```python
from build123d import *

# Parameters (mm, degrees)
F0_R     = 2.032
F0_R_2   = 2.027946
F0_R_3   = 6.35
F1_DEPTH = 6.35


with BuildPart() as f1:
    # F0 (on Top) → F1 (new body)
    with BuildSketch(Plane.XY):
        with BuildLine():
            Line((-170.272195, -49.641607), (-163.925477, -49.641607))
            ThreePointArc((-163.925477, -49.641607), (-140.909058, -31.963569), (-132.186283, -4.28358))
            Line((-132.186283, -4.28358), (-132.186283, -2.299813))
            Line((-132.186283, -2.299813), (-132.186283, 29.155357))
            ThreePointArc((-132.186283, 29.155357), (-133.837078, 32.141068), (-137.035743, 33.327715))
            Line((-137.035743, 33.327715), (-148.047195, 33.327715))
            Line((-148.047195, 33.327715), (-148.047195, 34.918903))
            Line((-148.047195, 34.918903), (-186.147195, 34.918903))
            Line((-186.147195, 34.918903), (-186.147195, 33.327715))
            Line((-186.147195, 33.327715), (-197.693917, 33.327715))
            Line((-197.693917, 33.327715), (-198.24493, 33.327715))
            ThreePointArc((-198.24493, 33.327715), (-201.203656, 31.805681), (-202.114563, 28.605541))
            Line((-202.114563, 28.605541), (-202.114563, 13.871952))
            Line((-202.114563, 13.871952), (-246.486589, 13.871952))
            Line((-246.486589, 13.871952), (-246.486589, -49.641607))
            Line((-246.486589, -49.641607), (-240.805238, -49.641607))
            Line((-240.805238, -49.641607), (-170.272195, -49.641607))
        make_face()
        with Locations((-234.114588, -44.87283)):
            Circle(F0_R, mode=Mode.SUBTRACT)
        with Locations((-167.098836, -46.955632)):
            Circle(F0_R, mode=Mode.SUBTRACT)
        with Locations((-167.098836, -41.466439)):
            Circle(F0_R_2, mode=Mode.SUBTRACT)
        with Locations((-233.186065, -3.547357)):
            Circle(F0_R_3, mode=Mode.SUBTRACT)
        with Locations((-197.969424, 21.535357)):
            Circle(F0_R, mode=Mode.SUBTRACT)
        with Locations((-197.969424, 29.155357)):
            Circle(F0_R, mode=Mode.SUBTRACT)
        with Locations((-167.097195, -3.291697)):
            Circle(F0_R_3, mode=Mode.SUBTRACT)
        with Locations((-137.035743, 21.535357)):
            Circle(F0_R, mode=Mode.SUBTRACT)
        with Locations((-137.035743, 29.155357)):
            Circle(F0_R, mode=Mode.SUBTRACT)
        with BuildLine():
            Line((-132.186283, -2.299813), (-132.186283, -4.28358))
            ThreePointArc((-132.186283, -4.28358), (-132.172195, -3.291697), (-132.186283, -2.299813))
        make_face()
        with BuildLine():
            ThreePointArc((-197.693917, 33.327715), (-197.969424, 33.336801), (-198.24493, 33.327715))
            Line((-198.24493, 33.327715), (-197.693917, 33.327715))
        make_face()
    extrude(amount=F1_DEPTH)


solid = f1.part
```
CAD build for the part. Positions are in the model's coordinates, mm. A direction names the side the tool comes from. Round coordinates to 2 decimals unless told otherwise and drop trailing zeros. Write each loop counter-clockwise with the first axis right and the second up, starting at its lowest first coordinate (ties: lowest second). Pieces come first, ordered by that corner, then holes. Notation, with made-up numbers: M 23.5,82 L 45.5,82 A13 ccw 45.5,92 Z; hole C 68,-25.5 d3. An arc over 180 degrees is marked long. One line per question, with ' | ' between items.
1. Cut at D-D on x = -217. Write the cut outline in (y, z).
Working result:
outline: M -49.64,0 L 13.87,0 L 13.87,6.35 L -49.64,6.35 Z
2. Cut at B-B on x = -230.5. Write the cut outline in (y, z).
Working result:
outline: M -49.64,0 L -9.3,0 L -9.3,6.35 L -49.64,6.35 Z; M 2.21,0 L 13.87,0 L 13.87,6.35 L 2.21,6.35 Z
3. Cut at A-A on y = -6.5. Write the cut outline in (x, z), and give its area (3 significant figures).
Working result:
outline: M -246.49,0 L -238.81,0 L -238.81,6.35 L -246.49,6.35 Z; M -227.56,0 L -172.58,0 L -172.58,6.35 L -227.56,6.35 Z; M -161.62,0 L -132.24,0 L -132.24,6.35 L -161.62,6.35 Z | area: 584 mm2
4. Probe L1, parallel to X at y = -6, z = 4.25; L2, parallel to Y at x = -168, z = 3.5; L3, parallel to X at y = 11.5, z = 0.5. List the from-to ranges inside material, lowest first. Write a range as from..to.
Working result:
L1: -246.49..-239.04, -227.33..-172.84, -161.35..-132.22 | L2: -49.64..-48.78, -45.13..-43.28, -39.65..-9.58, 2.99..34.92 | L3: -246.49..-132.19
5. Which spindle directions (+Z, -Z, +X, -X, +Y, -Y) get a long thin tool onto all of the face, cutting with end or side? Do faces 4 (the flat face through (-142, 33.328, 3)), 5 (the flat face through (-224, 13.872, 3)), 6 (the cylindrical face through (-239.53, -3.27, 3.13)). Say none if no direction does.
Working result:
face 4: +Z, -Z, +X, +Y | face 5: +Z, -Z, -X, +Y | face 6: +Z, -Z
6. Pin check, flat tips, straight feed: pin 1 Ø3 at (y, z) = (11, 2.5) entering from +X; pin 2 Ø1.9 at (x, z) = (-144, 4) entering from +Y; pin 3 Ø3.5 at (x, y) = (-167.1, -46.96) entering from -Z; pin 4 Ø0.8 at (y, z) = (34, 4) entering from -X. Stop position of each tip, or through.
Working result:
pin 1: x = -132.19 | pin 2: y = 33.33 | pin 3: through | pin 4: x = -186.15
7. Mould opens along Y. For faces 1 (the cylindrical face through (-133.8, 32.11, 3.13)), 2 (the cylindrical face through (-138.65, 20.3, 3.13)), 3 (the flat face through (-190, -7, 6.35)) say: pulls with the +Y half, pulls with the -Y half, needs draft (parallel to the pull), parting line crosses it, or undercut.
Working result:
face 1: pulls with the +Y half | face 2: undercut | face 3: needs draft
8. Cut at C-C on z = 2.25. Count the separate pieces of the cut face and the enclosed holes in it, and give its area (3 significant figures).
Working result:
separate pieces: 1 | enclosed holes: 9 | area: 7,940 mm2
